```python
from build123d import *

# Parameters (mm, degrees)
SKETCH1_R           = 4.5
BOSS_EXTRUDE1_DEPTH = 8
CHAMFER1_SIZE       = 1


with BuildPart() as part:
    # Sketch1 → Boss-Extrude1 (new body)
    with BuildSketch(Plane.XY):
        with BuildLine():
            Line((0, 9), (102, 9))
            ThreePointArc((102, 9), (111, 0), (102, -9))
            Line((102, -9), (0, -9))
            ThreePointArc((0, -9), (-9, 0), (0, 9))
        make_face()
        Circle(SKETCH1_R, mode=Mode.SUBTRACT)
        with Locations((102, 0)):
            Circle(SKETCH1_R, mode=Mode.SUBTRACT)
    extrude(amount=BOSS_EXTRUDE1_DEPTH)

    # Chamfer1
    chamfer1_edges = [part.edges().sort_by_distance(p)[0] for p in [
        (-4.5, 0, 8),
        (97.5, 0, 8),
    ]]
    chamfer(chamfer1_edges, length=CHAMFER1_SIZE)


solid = part.part
```
Input: part model. Units: mm. Frame: model coordinates. Coordinates: 2 decimals unless noted, no trailing zeros. Loops run counter-clockwise (first coordinate to the right, second up) from the corner with the lowest first, then second, coordinate; pieces in that order, holes last. Notation, with made-up numbers: M -32.5,54 L -27.5,54 A14 ccw -27.5,65 Z; hole C -25.75,51.5 d2. An arc over 180 degrees is marked long. One line per item, written item: value.
(1) Pull-direction query (X, two-part tool) for faces 1 (the cylindrical face through (97.504, 0.198, 3.451)), 2 (the cylindrical face through (-0.59, 4.46, 3.45)), 3 (the flat face through (50, 9, 4)), 4 (the cylindrical face through (-9, 0, 4)); classes: +X half, -X half, draft (parallel to the pull), parting line (faces both ways), or undercut.
Filled in:
face 1: undercut
face 2: undercut
face 3: draft
face 4: -X half
(2) Pin query (flat end, axial travel): pin 1 (1 mm diameter, centred on x = 3.5, y = -1.5, fed in from +Z); pin 2 (10.5 mm diameter, centred on x = 0, y = 0, fed in from +Z); pin 3 (1.5 mm diameter, centred on y = -5, z = 4.5, fed in from -X). Return the tip coordinate at first contact, or that it passes through.
Filled in:
pin 1: through
pin 2: z = 7.75
pin 3: x = -7.93
(3) Section A-A (y = 0). Output: boundary loops of the cut face in (x, z), and give its area (3 significant figures).
Filled in:
outline: M -9,0 L -4.5,0 L -4.5,7 L -5.5,8 L -9,8 Z; M 4.5,0 L 97.5,0 L 97.5,7 L 96.5,8 L 5.5,8 L 4.5,7 Z; M 106.5,0 L 111,0 L 111,8 L 107.5,8 L 106.5,7 Z
area: 814 mm^2
(4) Section C-C (y = -7). Output: boundary loops of the cut face in (x, z), and give its area (3 significant figures).
Filled in:
outline: M -5.66,0 L 107.66,0 L 107.66,8 L -5.66,8 Z
area: 907 mm^2
(5) Section B-B (z = 5.5). Output: boundary loops of the cut face in (x, y).
Filled in:
outline: M 0,-9 L 102,-9 A9 ccw 102,9 L 0,9 A9 ccw Z; hole C 0,0 d9; hole C 102,0 d9
(6) Line query: line 1 along X through (y, z) = (1.25, 6); line 2 along X through (y, z) = (-3.25, 7); line 3 along Y through (x, z) = (3.5, 1.25). Output: solid intervals per line, ascending. Write a range as from..to.
Filled in:
line 1: -8.91..-4.32, 4.32..97.68, 106.32..110.91
line 2: -8.39..-3.11, 3.11..98.89, 105.11..110.39
line 3: -9..-2.83, 2.83..9
